Input: dimensioned drawing with shaded views. Units: mm. Origin: part minimum x, y, z. A direction names the side the tool comes from. Round coordinates to 2 decimals unless told otherwise and drop trailing zeros. Loops run counter-clockwise (first coordinate to the right, second up) from the corner with the lowest first, then second, coordinate; pieces in that order, holes last.
Item 1: Access query for the marked faces 1, 2 and 3. Directions: +Z, -Z, +X, -X, +Y, -Y. A direction counts if a zero-diameter tool reaches every point of the face in a straight line with its end or side. Return the directions, or none.
Item 2: Section query D-D on y = 4.5. Return loops of the section in (x, z), then the cut area to 3 significant figures.
Item 3: Section query A-A on z = 2.5. Return loops of the section in (x, y).
Item 4: Section query C-C on x = 19.75. Return loops of the section in (y, z).
Item 5: Ray query, L1, parallel to Z at x = 17.5, y = 2.4; L2, parallel to X at y = 1.4, z = 1.4; L3, parallel to Y at x = 19.75, z = 4.7. Return the intervals inside material, ascending.
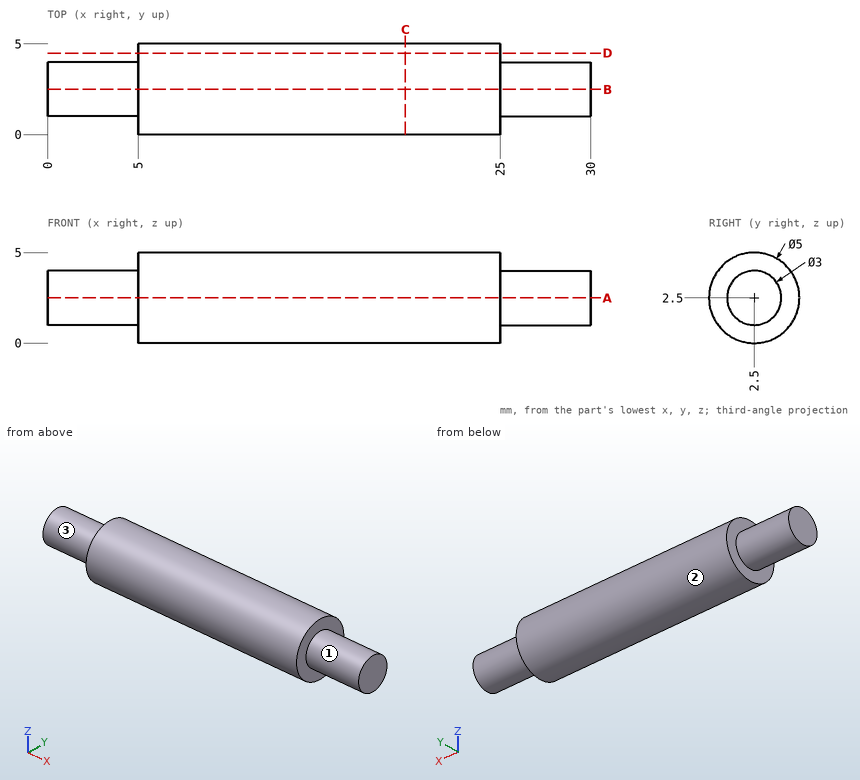
Data:
1. face 1: +X
1. face 2: +X, -X
1. face 3: -X
2. outline: (5, 1) - (25, 1) - (25, 4) - (5, 4) - close
2. area: 60.0 mm2
3. outline: (0, 1) - (5, 1) - (5, 0) - (25, 0) - (25, 1) - (30, 1) - (30, 4) - (25, 4) - (25, 5) - (5, 5) - (5, 4) - (0, 4) - close
4. outline: circle Ø5 at (2.5, 2.5)
5. L1: z = 0 to 5
5. L2: x = 5 to 25
5. L3: y = 1.31 to 3.69
